from build123d import *

# Parameters (mm, degrees)
F1_DEPTH = 300
F2_R     = 31
F3_DEPTH = 20
F4_R     = 10
F5_DEPTH = 20


with BuildPart() as f1:
    # F0 (on Front) → F1 (new body)
    with BuildSketch(Plane.XZ):
        Polygon((165, 0), (0, 0), (0, -170), (20, -170), (20, -20), (145, -20), (145, -320), (165, -320), (165, -20), align=None)
    extrude(amount=F1_DEPTH)

    # F2 (on face) → F3 (cut, through all)
    with BuildSketch(Plane(origin=(0, 0, 0), x_dir=(0, -1, 0), z_dir=(-1, 0, 0))):
        with Locations((150, -100)):
            Circle(F2_R)
    extrude(amount=-F3_DEPTH, mode=Mode.SUBTRACT)

    # F4 (on face) → F5 (cut, through all)
    with BuildSketch(Plane.YZ.offset(165)):
        with Locations((-150, -60)):
            Circle(F4_R)
        with Locations((-245.105652, -129.098301)):
            Circle(F4_R)
        with Locations((-208.778525, -240.901699)):
            Circle(F4_R)
        with Locations((-91.221475, -240.901699)):
            Circle(F4_R)
        with Locations((-54.894348, -129.098301)):
            Circle(F4_R)
    extrude(amount=-F5_DEPTH, mode=Mode.SUBTRACT)


solid = f1.part
Can you work these out from the model? Positions are in its coordinate system, mm. A direction names the side the tool comes from. Round coordinates to 2 decimals unless told otherwise and drop trailing zeros. Loops run counter-clockwise (first coordinate to the right, second up) from the corner with the lowest first, then second, coordinate; pieces in that order, holes last. Notation, with made-up numbers: (-19, 71.5) - (35, 71.5) arc R23 ccw to (35, 99.5) - close; hole circle Ø1 at (-8, 75). An arc over 180 degrees is marked (long way). Answer in a Markdown table with one row per item. Add a question column.
Q1. I want a section at A-A on z = -100. List the corners of the cut face in (x, y) for me.
Q2. I want a section at D-D on x = 43.5. List the corners of the cut face in (y, z) for me, and give its area (3 significant figures).
Q3. I want a section at C-C on z = -60. List the corners of the cut face in (x, y) for me, and give its area (3 significant figures).
Q4. For pin 1 Ø5 at (x, y) = (48, -105.5) entering from -Z; pin 2 Ø18 at (y, z) = (-54.89, -129.1) entering from +X; pin 3 Ø6 at (x, y) = (14.5, -127) entering from -Z, each with a flat end and sliding along its axis, tell me the tip position at first contact or that it passes through.
Q5. I need wall thicknesses on L1, parallel to X at y = -147, z = -131; L2, parallel to Z at x = 59.5, y = -204.5; L3, parallel to X at y = -14, z = -272. Which ranges of each line are inside material? Lowest first, please.
Q6. Which directions (+Z, -Z, +X, -X, +Y, -Y) give clear straight access to the entire face, cutting with the end or side of a thin tool? Please do faces 1 (the flat face through (20, -148, -63)), 2 (the cylindrical face through (155.14, -56.196, -119.183)), 3 (the cylindrical face through (9.86, -119.03, -98.64)).
Q7. We'd pull the mould along Y, two halves only. Please class faces 4 (the cylindrical face through (155.14, -235.57, -126.09)), 5 (the flat face through (149, 0, -112)), 6 (the flat face through (155, -148, -320)): pulls with the +Y half, pulls with the -Y half, needs draft (parallel to the pull), parting line crosses it, or undercut.
Q8. I want a section at B-B on y = -150. List the corners of the cut face in (x, z) for me.
A:
| question | item | result |
|---|---|---|
| 1 | outline | (0, -300) - (20, -300) - (20, -181) - (0, -181) - close; (0, -119) - (20, -119) - (20, 0) - (0, 0) - close; (145, -300) - (165, -300) - (165, 0) - (145, 0) - close |
| 2 | outline | (-300, -20) - (0, -20) - (0, 0) - (-300, 0) - close |
| 2 | area | 6,000 mm^2 |
| 3 | outline | (0, -300) - (20, -300) - (20, 0) - (0, 0) - close; (145, -300) - (165, -300) - (165, -160) - (145, -160) - close; (145, -140) - (165, -140) - (165, 0) - (145, 0) - close |
| 3 | area | 11,600 mm^2 |
| 4 | pin 1 | z = -20 |
| 4 | pin 2 | x = 20 |
| 4 | pin 3 | z = -170 |
| 5 | L1 | 0 to 20, 145 to 165 |
| 5 | L2 | -20 to 0 |
| 5 | L3 | 145 to 165 |
| 6 | face 1 | -Z, +Y, -Y |
| 6 | face 2 | +X |
| 6 | face 3 | -X |
| 7 | face 4 | undercut |
| 7 | face 5 | pulls with the +Y half |
| 7 | face 6 | needs draft |
| 8 | outline | (0, -170) - (20, -170) - (20, -131) - (0, -131) - close; (0, -69) - (20, -69) - (20, -20) - (145, -20) - (145, -50) - (165, -50) - (165, 0) - (0, 0) - close; (145, -320) - (165, -320) - (165, -70) - (145, -70) - close |
